```python
from build123d import *

# Parameters (mm, degrees)
SKETCH1_R           = 9.525
BOSS_EXTRUDE1_DEPTH = 304.8
DOME1_FACE_RADIUS   = 9.525
DOME1_HEIGHT        = 9.525


# Read off the part's stored shape, not the designer's step: Shell1
with BuildPart() as part:
    # Sketch1 → Boss-Extrude1 (new body)
    with BuildSketch(Plane(origin=(0, 0, 0), x_dir=(0, 0, -1), z_dir=(1, 0, 0))):
        Circle(SKETCH1_R)
    extrude(amount=-BOSS_EXTRUDE1_DEPTH)

    # Dome1: a dome of height H over a round flat face of radius A is a cap of a sphere of radius (A * A + H * H) / (2 * H)
    dome1_r = (DOME1_FACE_RADIUS * DOME1_FACE_RADIUS + DOME1_HEIGHT * DOME1_HEIGHT) / (2 * DOME1_HEIGHT)
    dome1_base = Plane((-304.8, 0, 0), z_dir=(-1, 0, 0))
    with Locations(dome1_base.offset(DOME1_HEIGHT - dome1_r)):
        dome1_ball = Sphere(dome1_r, mode=Mode.PRIVATE)
    add(split(dome1_ball, bisect_by=dome1_base, keep=Keep.TOP, mode=Mode.PRIVATE))

    # Shell1 outline → Shell1 (revolve, cut)
    with BuildSketch(Plane.YX):
        with BuildLine():
            ThreePointArc((0, -311.785), (4.939140869, -309.739140864), (6.985, -304.799999993))
            Line((6.985, -304.799999993), (6.985, 0))
            Line((6.985, 0), (0, 0))
            Line((0, 0), (0, -311.785))
        make_face()
    revolve(axis=Axis((0, 0, 0), (1, 0, 0)), mode=Mode.SUBTRACT)


solid = part.part
```
Verification items for the finished model (mm, model axes). Give positions to 0.01 mm unless a question says otherwise; leave off trailing zeros. Loops run counter-clockwise (first coordinate to the right, second up) from the corner with the lowest first, then second, coordinate; pieces in that order, holes last.
1. Section check C-C, the plane x = -60. Enter the section's corners in (y, z) (3 decimals), then the cut area to 3 significant figures.
2. Mould release check, pull along Z, two halves, no side actions. Record for faces 1 (the cylindrical face through (-150.266, -0.909, 6.926)), 2 (the cylindrical face through (-150.266, -5.796, 7.559)), 3 (the flat face through (0, 7.1, 0.8)): released by +Z, released by -Z, zero draft, split by the parting line, or undercut.
3. Thickness scan on line 1 (Z direction, x = -206, y = -0.5); line 2 (Y direction, x = -158, z = -4.75); line 3 (Y direction, x = -253.5, z = -3.5). Record the ranges inside material, lowest first.
4. Section check A-A, the plane z = 0. Enter the section's corners in (x, y) (3 decimals).
5. Go/stop test with flat-tipped pins: pin 1 Ø1 at (x, z) = (-57, -2) entering from -Y; pin 2 Ø6 at (y, z) = (1, -5) entering from -X; pin 3 Ø2 at (x, y) = (-207, 7) entering from -Z. Record where each tip stops, or that it passes through.
Geometry says:
1. outline: circle Ø19.05 at (0, 0); hole circle Ø13.97 at (0, 0)
1. area: 132 mm2
2. face 1: undercut
2. face 2: split by the parting line
2. face 3: zero draft
3. line 1: z = -9.51 to -6.97, 6.97 to 9.51
3. line 2: y = -8.26 to -5.12, 5.12 to 8.26
3. line 3: y = -8.86 to -6.04, 6.04 to 8.86
4. outline: (-304.8, -9.525) - (0, -9.525) - (0, -6.985) - (-304.8, -6.985) arc R6.985 cw to (-304.8, 6.985) - (0, 6.985) - (0, 9.525) - (-304.8, 9.525) arc R9.525 ccw to start
5. pin 1: stops at y = -9.41
5. pin 2: stops at x = -314.09
5. pin 3: stops at z = -7.4
